Geometry: final body of the model. Coordinates: model frame, mm. Face numbers are marked on the shaded views. A direction names the side the tool comes from. Give positions to 0.01 mm unless a question says otherwise; leave off trailing zeros. Write each loop counter-clockwise with the first axis right and the second up, starting at its lowest first coordinate (ties: lowest second). Pieces come first, ordered by that corner, then holes. Notation, with made-up numbers: (-23, -4.5) - (-6, -4.5) arc R24 ccw to (-6, 16.5) - close; hole circle Ø1 at (25.25, -0.5). An arc over 180 degrees is marked (long way). One line per question, with ' | ' between items. Start each with the question number.
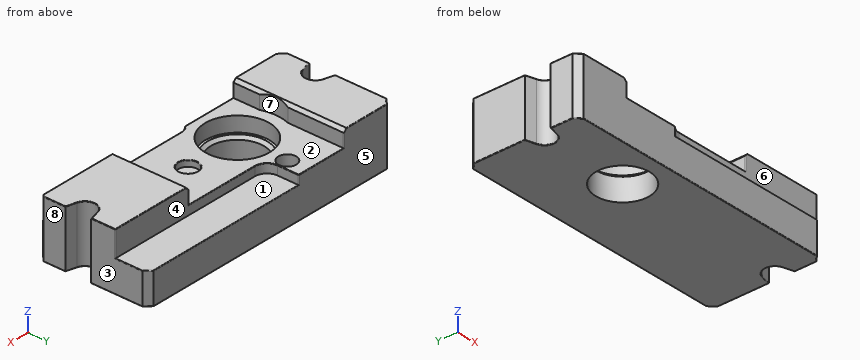
```python
from build123d import *

# Parameters (mm, degrees)
F0_R     = 8.9
F3_DEPTH = 13.5
F0_W     = 27.7
F0_H     = 1.2
F0_H_2   = 11
F4_DEPTH = 10.5
F2_R     = 10.7
F5_DEPTH = 5
F2_R_2   = 3.25
F6_DEPTH = 2
F2_R_3   = 3
F7_DEPTH = 6
F8_DEPTH = 5.5
F9_SIZE  = 1
F10_SIZE = 2
F11_R    = 0.2


with BuildPart() as f3:
    # F0 (on Top) → F3 (new body)
    with BuildSketch(Plane.XY):
        with BuildLine():
            Line((0, 9.2066603875), (0, 0))
            Line((0, 0), (18.3, 0))
            Line((18.3, 0), (18.3, 8.7502631652))
            ThreePointArc((18.3, 8.7502631652), (17.5, 13.5), (18.3, 18.2497368348))
            Line((18.3, 18.2497368348), (18.3, 36.8))
            Line((18.3, 36.8), (0, 36.8))
            Line((0, 36.8), (0, 17.7933396125))
            Line((0, 17.7933396125), (3.4058666579, 16.880740392))
            ThreePointArc((3.4058666579, 16.880740392), (6, 13.5), (3.4058666579, 10.119259608))
            Line((3.4058666579, 10.119259608), (0, 9.2066603875))
        make_face()
        with BuildLine():
            Line((18.3, 8.7502631652), (18.3, 0))
            Line((18.3, 0), (36.4434286286, 0))
            ThreePointArc((36.4434286286, 0), (37.7508066615, 0.8878177829), (39.3, 1.2))
            Line((39.3, 1.2), (64.3, 1.2))
            Line((64.3, 1.2), (64.3, 25.8))
            Line((64.3, 25.8), (39.3, 25.8))
            ThreePointArc((39.3, 25.8), (36.4715728753, 26.9715728753), (35.3, 29.8))
            Line((35.3, 29.8), (35.3, 36.8))
            Line((35.3, 36.8), (18.3, 36.8))
            Line((18.3, 36.8), (18.3, 18.2497368348))
            ThreePointArc((18.3, 18.2497368348), (17.5, 13.5), (18.3, 8.7502631652))
        make_face()
        with Locations((32, 13.5)):
            Circle(F0_R, mode=Mode.SUBTRACT)
        with BuildLine():
            Line((64.3, 25.8), (64.3, 1.2))
            Line((64.3, 1.2), (92, 1.2))
            Line((92, 1.2), (92, 9.2066603875))
            Line((92, 9.2066603875), (88.5941333421, 10.119259608))
            ThreePointArc((88.5941333421, 10.119259608), (86, 13.5), (88.5941333421, 16.880740392))
            Line((88.5941333421, 16.880740392), (92, 17.7933396125))
            Line((92, 17.7933396125), (92, 25.8))
            Line((92, 25.8), (64.3, 25.8))
        make_face()
    extrude(amount=F3_DEPTH)

    # F0 (on Top) → F4 (join)
    with BuildSketch(Plane.XY):
        with Locations((78.15, 0.6)):
            Rectangle(F0_W, F0_H)
        with BuildLine():
            ThreePointArc((39.3, 1.2), (37.7508066615, 0.8878177829), (36.4434286286, 0))
            Line((36.4434286286, 0), (64.3, 0))
            Line((64.3, 0), (64.3, 1.2))
            Line((64.3, 1.2), (39.3, 1.2))
        make_face()
        with BuildLine():
            Line((39.3, 25.8), (64.3, 25.8))
            Line((64.3, 25.8), (64.3, 36.8))
            Line((64.3, 36.8), (35.3, 36.8))
            Line((35.3, 36.8), (35.3, 29.8))
            ThreePointArc((35.3, 29.8), (36.4715728753, 26.9715728753), (39.3, 25.8))
        make_face()
        with Locations((78.15, 31.3)):
            Rectangle(F0_W, F0_H_2)
    extrude(amount=F4_DEPTH)

    # F2 (on offset) → F5 (cut)
    with BuildSketch(Plane.XY.offset(13.5)):
        with Locations((32, 13.5)):
            Circle(F2_R)
    extrude(amount=-F5_DEPTH, mode=Mode.SUBTRACT)

    # F2 (on offset) → F6 (cut)
    with BuildSketch(Plane.XY.offset(13.5)):
        with Locations((50.6, 13.5)):
            Circle(F2_R_2)
    extrude(amount=-F6_DEPTH, mode=Mode.SUBTRACT)

    # F2 (on offset) → F7 (cut)
    with BuildSketch(Plane.XY.offset(13.5)):
        with Locations((32, 30.1)):
            Circle(F2_R_3)
    extrude(amount=-F7_DEPTH, mode=Mode.SUBTRACT)

    # F2 (on offset) → F8 (join)
    with BuildSketch(Plane.XY.offset(13.5)):
        with BuildLine():
            Line((18.3, 0), (18.3, 8.7502631652))
            ThreePointArc((18.3, 8.7502631652), (17.5, 13.5), (18.3, 18.2497368348))
            Line((18.3, 18.2497368348), (18.3, 36.8))
            Line((18.3, 36.8), (0, 36.8))
            Line((0, 36.8), (0, 17.7933396125))
            Line((0, 17.7933396125), (3.4058666579, 16.880740392))
            ThreePointArc((3.4058666579, 16.880740392), (6, 13.5), (3.4058666579, 10.119259608))
            Line((3.4058666579, 10.119259608), (0, 9.2066603875))
            Line((0, 9.2066603875), (0, 0))
            Line((0, 0), (18.3, 0))
        make_face()
        with BuildLine():
            Line((92, 17.7933396125), (92, 25.8))
            Line((92, 25.8), (64.3, 25.8))
            Line((64.3, 25.8), (64.3, 1.2))
            Line((64.3, 1.2), (92, 1.2))
            Line((92, 1.2), (92, 9.2066603875))
            Line((92, 9.2066603875), (88.5941333421, 10.119259608))
            ThreePointArc((88.5941333421, 10.119259608), (86, 13.5), (88.5941333421, 16.880740392))
            Line((88.5941333421, 16.880740392), (92, 17.7933396125))
        make_face()
    extrude(amount=F8_DEPTH)

    # F9
    f9_edges = [f3.edges().sort_by_distance(p)[0] for p in [
        (23.1, 13.5, 8.5),
        (18.3, 27.524868, 19),
        (64.3, 13.5, 19),
    ]]
    chamfer(f9_edges, length=F9_SIZE)

    # F10
    f10_edges = [f3.edges().sort_by_distance(p)[0] for p in [
        (92, 0, 5.25),
        (92, 36.8, 5.25),
        (0, 36.8, 9.5),
        (0, 0, 9.5),
    ]]
    chamfer(f10_edges, length=F10_SIZE)

    # F11
    f11_edges = [f3.edges().sort_by_distance(p)[0] for p in [
        (1, 1, 19),
        (0, 5.60333, 19),
        (1.702933, 9.66296, 19),
        (6, 13.5, 19),
        (0, 26.29667, 19),
        (1.702933, 17.33704, 19),
        (1, 35.8, 19),
        (9.65, 36.8, 19),
        (17.8, 36.8, 18.5),
        (18.3, 36.8, 15.75),
        (26.8, 36.8, 13.5),
        (35.3, 36.8, 12),
        (62.65, 36.8, 10.5),
        (91, 35.8, 10.5),
        (92, 30.3, 10.5),
        (92, 25.8, 14.75),
        (78.65, 25.8, 19),
        (78.25, 1.2, 19),
        (91.6, 1.6, 19),
        (92, 5.60333, 19),
        (90.297067, 9.66296, 19),
        (86, 13.5, 19),
        (92, 21.79667, 19),
        (64.3, 1.2, 15.75),
        (51.8, 1.2, 13.5),
        (27.371714, 0, 13.5),
        (18.3, 0, 15.75),
        (17.8, 0, 18.5),
        (9.65, 0, 19),
        (64.3, 25.8, 15.75),
        (64.8, 25.8, 18.5),
        (51.8, 25.8, 13.5),
        (36.471573, 26.971573, 13.5),
        (35.3, 33.3, 13.5),
        (46, 36.8, 0),
        (91, 35.8, 0),
        (92, 26.29667, 0),
        (90.297067, 17.33704, 0),
        (86, 13.5, 0),
        (92, 5.60333, 0),
        (91, 1, 0),
        (46, 0, 0),
        (1, 1, 0),
        (0, 5.60333, 0),
        (1.702933, 9.66296, 0),
        (1, 35.8, 0),
        (0, 26.29667, 0),
        (47.35, 13.5, 13.5),
    ]]
    fillet(f11_edges, radius=F11_R)


solid = f3.part
```
1) Reachability of the marked faces 4, 5, 6, 7 and 8 from +Z, -Z, +X, -X, +Y, -Y: full face, straight path, thin tool, end or side. Return the list, or none.
2) Section D-D, the plane x = 69.5. Output: boundary loops of the cut face in (y, z).
3) First-contact query: pin 1 Ø10.5 at (x, y) = (29.5, 16.5) entering from +Z; pin 2 Ø4 at (x, z) = (72, 16.5) entering from -Y; pin 3 Ø8 at (y, z) = (14, 4.5) entering from +X; pin 4 Ø6.5 at (x, z) = (53.5, 16.5) entering from +Y. Flat tips, straight axial feed; report the tip coordinate or a pass-through.
4) Line query: L1, parallel to Y at x = 32, z = 9.9; L2, parallel to X at y = 19, z = 16.5; L3, parallel to Y at x = 32, z = 4.25. Output: solid intervals per line, ascending.
5) Pull-direction query (X, two-part tool) for the marked faces 1, 2 and 3; classes: +X half, -X half, draft (parallel to the pull), parting line (faces both ways), or undercut.
6) Section B-B, the plane x = 32. Output: boundary loops of the cut face in (y, z).
7) Section C-C, the plane z = 4. Output: boundary loops of the cut face in (x, y), plus the area to 3 significant figures.
Answer key:
1) face 4: +Z, +X, +Y | face 5: +Z, -Z, +X, -X, +Y | face 6: +Z, +X, -Y | face 7: +Z | face 8: +Z, -Z, +X, +Y, -Y
2) outline: (0, 0.2) arc R0.2 ccw to (0.2, 0) - (36.6, 0) arc R0.2 ccw to (36.8, 0.2) - (36.8, 10.3) arc R0.2 ccw to (36.6, 10.5) - (25.8, 10.5) - (25.8, 18.8) arc R0.2 ccw to (25.6, 19) - (1.4, 19) arc R0.2 ccw to (1.2, 18.8) - (1.2, 10.5) - (0, 10.5) - close
3) pin 1: z = 7.76 | pin 2: y = 1.2 | pin 3: x = 92 | pin 4: y = 25.8
4) L1: 0 to 2.8, 24.2 to 27.1, 33.1 to 36.8 | L2: 0 to 18.3, 64.3 to 92 | L3: 0 to 4.6, 22.4 to 36.8
5) face 1: draft | face 2: undercut | face 3: +X half
6) outline: (0, 0.2) arc R0.2 ccw to (0.2, 0) - (4.6, 0) - (4.6, 7.5) - (3.6, 8.5) - (2.8, 8.5) - (2.8, 13.5) - (0.2, 13.5) arc R0.2 ccw to (0, 13.3) - close; (22.4, 0) - (36.6, 0) arc R0.2 ccw to (36.8, 0.2) - (36.8, 13.3) arc R0.2 ccw to (36.6, 13.5) - (33.1, 13.5) - (33.1, 7.5) - (27.1, 7.5) - (27.1, 13.5) - (24.2, 13.5) - (24.2, 8.5) - (23.4, 8.5) - (22.4, 7.5) - close
7) outline: (0, 2) - (2, 0) - (90, 0) - (92, 2) - (92, 9.21) - (88.59, 10.12) arc R3.5 cw to (88.59, 16.88) - (92, 17.79) - (92, 34.8) - (90, 36.8) - (2, 36.8) - (0, 34.8) - (0, 17.79) - (3.41, 16.88) arc R3.5 cw to (3.41, 10.12) - (0, 9.21) - close; hole circle Ø17.8 at (32, 13.5) | area: 3,050 mm^2
